For this review, take the finished solid that the model builds, in its own axes (mm). A direction names the side the tool comes from. Give positions to 0.01 mm unless a question says otherwise; leave off trailing zeros. Loops run counter-clockwise (first coordinate to the right, second up) from the corner with the lowest first, then second, coordinate; pieces in that order, holes last.
```python
from build123d import *

# Parameters (mm, degrees)
F0_R          = 11.0236
F0_R_2        = 5.842
F0_R_3        = 3.9624
F1_DEPTH      = 6.985
F2_R          = 0.635
F3_R          = 5.9436
F3_R_2        = 3.9624
F4_DEPTH      = 0.254
F4_DEPTH_BACK = 7.239


with BuildPart() as f1:
    # F0 (on Top) → F1 (new body)
    with BuildSketch(Plane.XY):
        Circle(F0_R)
        Circle(F0_R_2, mode=Mode.SUBTRACT)
        Circle(F0_R_2)
        Circle(F0_R_3, mode=Mode.SUBTRACT)
    extrude(amount=F1_DEPTH)

    # F2
    f2_edges = [f1.edges().sort_by_distance(p)[0] for p in [
        (-11.0236, 0, 0),
        (-11.0236, 0, 6.985),
    ]]
    fillet(f2_edges, radius=F2_R)

    # F3 (on face) → F4 (join, two sides)
    with BuildSketch(Plane.XY.offset(6.985)) as f4_sk:
        Circle(F3_R)
        Circle(F3_R_2, mode=Mode.SUBTRACT)
    extrude(amount=F4_DEPTH)
    extrude(f4_sk.sketch, amount=-F4_DEPTH_BACK)


solid = f1.part
```
Item 1: For L1, parallel to Y at x = 0, z = 7.1; L2, parallel to Z at x = -8.25, y = -1 (3 decimals); L3, parallel to X at y = -3.25, z = 6.75, list the stretches that pass through material, from the lowest coordinate up.
Answer:
L1: y = -5.94 to -3.96, 3.96 to 5.94
L2: z = 0 to 6.985
L3: x = -10.39 to -2.27, 2.27 to 10.39
Item 2: Tool access review of faces 1 (the flat face through (4.5, -4.5, 6.985)), 2 (the flat face through (4.5, -4.5, 0)), 3 (the flat face through (4, -1, 7.239)): name each direction out of +Z, -Z, +X, -X, +Y, -Y from which nothing blocks a thin tool from reaching the whole face with its end or side.
Answer:
face 1: +Z
face 2: -Z
face 3: +Z, +X, -X, +Y, -Y
Item 3: Take a section at A-A on x = 0. Give the boundary of the cut face in (y, z) (3 decimals), and give its area (3 significant figures).
Answer:
outline: (-11.024, 0.635) arc R0.635 ccw to (-10.389, 0) - (-5.944, 0) - (-5.944, -0.254) - (-3.962, -0.254) - (-3.962, 7.239) - (-5.944, 7.239) - (-5.944, 6.985) - (-10.389, 6.985) arc R0.635 ccw to (-11.024, 6.35) - close; (3.962, -0.254) - (5.944, -0.254) - (5.944, 0) - (10.389, 0) arc R0.635 ccw to (11.024, 0.635) - (11.024, 6.35) arc R0.635 ccw to (10.389, 6.985) - (5.944, 6.985) - (5.944, 7.239) - (3.962, 7.239) - close
area: 100 mm2
Item 4: Clearance check with a flat-ended pin moving along its axis: pin 1 Ø1.5 at (x, z) = (6, 0.5) entering from -Y. State where the tip first meets the part, or that it passes through.
Answer:
pin 1: stops at y = -9.69
Item 5: Take a section at C-C on z = 1.5. Give the boundary of the cut face in (x, y), and give its area (3 significant figures).
Answer:
outline: circle Ø22.05 at (0, 0); hole circle Ø7.92 at (0, 0)
area: 332 mm2
